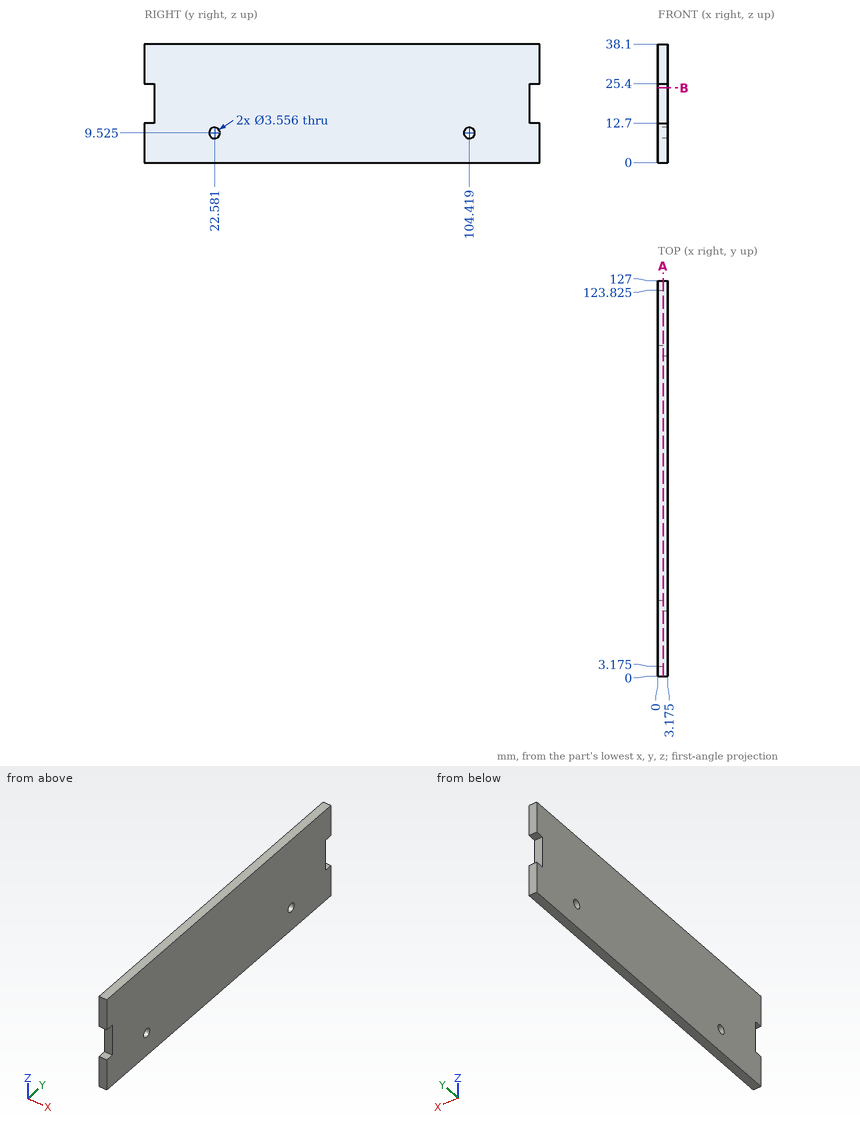
Drawing for the job (mm, zero at the part's lowest x, y, z). Give positions to 0.01 mm unless a question says otherwise; leave off trailing zeros. Loops run counter-clockwise (first coordinate to the right, second up) from the corner with the lowest first, then second, coordinate; pieces in that order, holes last.
(1) Band-saw the part on A-A (x = 1.75). Write the cut outline in (y, z) (1 decimal).
Return value:
outline: (0, 0) - (127, 0) - (127, 12.7) - (123.8, 12.7) - (123.8, 25.4) - (127, 25.4) - (127, 38.1) - (0, 38.1) - (0, 25.4) - (3.2, 25.4) - (3.2, 12.7) - (0, 12.7) - close; hole circle Ø3.6 at (22.6, 9.5); hole circle Ø3.6 at (104.4, 9.5)
(2) Drill centre lines: line 1 along Y through (x, z) = (2, 10) (1 decimal); line 2 along Y through (x, z) = (0.5, 17) (1 decimal). Where is each one in solid material? Low to high.
Return value:
line 1: y = 0 to 20.9, 24.3 to 102.7, 106.1 to 127
line 2: y = 3.2 to 123.8
(3) Band-saw the part on B-B (z = 24). Write the cut outline in (x, y) (1 decimal).
Return value:
outline: (0, 3.2) - (3.2, 3.2) - (3.2, 123.8) - (0, 123.8) - close
(4) Pin check, flat tips, straight feed: pin 1 (1.6 mm diameter, centred on x = 1, z = 20.5, fed in from -Y) (3 decimals); pin 2 (1 mm diameter, centred on x = 0.5, z = 13.5, fed in from +Y) (3 decimals). Stop position of each tip, or through.
Return value:
pin 1: stops at y = 3.175
pin 2: stops at y = 123.825
